```python
from build123d import *

# Parameters (mm, degrees)
F1_DEPTH = 101.6
F2_T     = -3.175
F3_R     = 3.175
F4_DEPTH = 25.4


with BuildPart() as f1:
    # F0 (on Right) → F1 (new body)
    with BuildSketch(Plane.YZ):
        Polygon((185.428325, -23.156608), (-195.571675, -23.156608), (-119.371675, -124.756608), (185.428325, -124.756608), align=None)
    extrude(amount=F1_DEPTH)

    # F2
    f2_openings = [f1.faces().sort_by_distance(p)[0] for p in [
        (50.8, -157.471675, -73.956608),
    ]]
    offset(amount=F2_T, openings=f2_openings)

    # F3 (on face) → F4 (cut)
    with BuildSketch(Plane(origin=(0, 0, -124.756608), x_dir=(1, 0, 0), z_dir=(0, 0, -1))):
        with Locations((25.4, 93.971675)):
            Circle(F3_R)
        with Locations((76.2, 93.971675)):
            Circle(F3_R)
        with Locations((25.4, -160.028325)):
            Circle(F3_R)
        with Locations((76.2, -160.028325)):
            Circle(F3_R)
    extrude(amount=-F4_DEPTH, mode=Mode.SUBTRACT)


solid = f1.part
```
Check sheet for the modelled part. Datum: model origin and axes. Units: mm. A direction names the side the tool comes from. Coordinates: 2 decimals unless noted, no trailing zeros. Write each loop counter-clockwise with the first axis right and the second up, starting at its lowest first coordinate (ties: lowest second). Pieces come first, ordered by that corner, then holes. Notation, with made-up numbers: M -24.5,-38.5 L 2.5,-38.5 A12 cw 2.5,-32.5 Z; hole C 59,20.25 d4. An arc over 180 degrees is marked long. Use one line per item in the form item = value.
Item 1: Sectioned sample at A-A, the plane y = 28.5. Record the cut outline in (x, z) (3 decimals).
Answer below:
outline = M 0,-124.757 L 101.6,-124.757 L 101.6,-23.157 L 0,-23.157 Z; hole M 3.175,-121.582 L 98.425,-121.582 L 98.425,-26.332 L 3.175,-26.332 Z
Item 2: Sectioned sample at B-B, the plane x = 47.5. Record the cut outline in (y, z), and give its area (3 significant figures).
Answer below:
outline = M -195.57,-23.16 L -193.19,-26.33 L 182.25,-26.33 L 182.25,-121.58 L -121.75,-121.58 L -119.37,-124.76 L 185.43,-124.76 L 185.43,-23.16 Z
area = 2,480 mm^2
Item 3: Release check for a two-part mould opening along Y. For faces 1 (the face through (50, 185.428, -75)), 2 (the face through (50, 182.253, -75)), 3 (the face through (28.428, 159.075, -123.191)), 4 (the face through (50, 31, -124.757)) record: pulls with the +Y half, pulls with the -Y half, needs draft (parallel to the pull), parting line crosses it, or undercut.
Answer below:
face_1 = pulls with the +Y half
face_2 = pulls with the -Y half
face_3 = undercut
face_4 = needs draft
Item 4: Gauge pin test, flat end, axial feed: pin 1 Ø2 at (x, y) = (51.5, -147) entering from -Z. Record the tip position at first contact, or that the pin passes through.
Answer below:
pin_1 = -26.33
Item 5: Sectioned sample at C-C, the plane z = -32. Record the cut outline in (x, y) (3 decimals), and give its area (3 significant figures).
Answer below:
outline = M 0,-188.939 L 3.175,-188.939 L 3.175,182.253 L 98.425,182.253 L 98.425,-188.939 L 101.6,-188.939 L 101.6,185.428 L 0,185.428 Z
area = 2,680 mm^2
Item 6: Set-up check for faces 5 (the face through (75.512, -90.872, -123.191)), 6 (the face through (101.6, -8, -73)), 7 (the face through (98.425, -8, -73)): record each of +Z, -Z, +X, -X, +Y, -Y from which the full face is reachable in a straight line by a thin tool's end or side.
Answer below:
face_5 = -Z
face_6 = +Z, -Z, +X, +Y, -Y
face_7 = -Y
Item 7: Material ranges on L1, parallel to Z at x = 79.5, y = 169; L2, parallel to X at y = 16, z = -46.5 (3 decimals); L3, parallel to Y at x = 76, z = -123, recorded low to high. Write a range as from..to.
Answer below:
L1 = -124.76..-121.58, -26.33..-23.16
L2 = 0..3.175, 98.425..101.6
L3 = -120.69..-97.14, -90.8..156.86, 163.2..185.43
